Input: part model. Units: mm. Frame: model coordinates. A direction names the side the tool comes from. Give positions to 0.01 mm unless a question says otherwise; leave off trailing zeros. Loops run counter-clockwise (first coordinate to the right, second up) from the corner with the lowest first, then second, coordinate; pieces in that order, holes last.
Autodesk Inventor part; units mm, degrees
ref_plane "YZ Plane" through (0, 0, 0) normal (1, 0, 0) x (0, 1, 0)
ref_plane "XZ Plane" through (0, 0, 0) normal (0, 1, 0) x (-1, 0, 0)
ref_plane "XY Plane" through (0, 0, 0) normal (0, 0, 1) x (1, 0, 0)
sketch "Sketch1" plane through (0, 0, 0) normal (0, 0, 1) x (1, 0, 0)
  line L0 (177.8, -0.9299) -> (0, -0.9299)
  line L1 (175.895, 75.2701) -> (177.8, 75.2701)
  line L2 (172.72, 5.08) -> (172.72, 72.0951)
  arc A0 (175.895, 75.2701) -> (172.72, 72.0951) centre (175.895, 72.0951) ccw
  line L3 (177.8, -0.9299) -> (177.8, 75.2701)
  line L4 (172.72, 5.08) -> (0, 5.08)
  line L5 (0, 5.08) -> (0, -0.9299)
  point P0 (172.72, 75.2701)
  dimension "d0" = 177.8
  dimension "d4" = 3.175
  dimension "d6" = 1.905
  dimension "d87" = 76.2
extrude "Extrusion1" add sketch "Sketch1" along normal blind 127
sketch "Sketch5" plane through (0, 5.08, 0) normal (0, 1, 0) x (1, 0, 0)
  line L0 (172.72, -127) -> (71.12, -127) construction
  line L1 (0, 0) -> (0, -127)
  line L2 (5.08, 0) -> (0, 0)
  arc A0 (0, 0) -> (66.04, -127) centre (174.6906, 10.1687) ccw
  line L3 (71.12, -127) -> (66.04, -127)
  line L4 (172.72, -127) -> (71.12, -127)
  line L5 (0, -127) -> (177.8, -127)
  line L6 (172.72, -127) -> (0, -127)
  dimension "d99" = 5.08
  dimension "d100" = 5.08
  dimension "d134" = 101.6
split body "Split2" sketch "Sketch5" result one side removed curves L2 A0 L3 removed pieces at (22.8484, 4.58, 104.8944)
sketch "Sketch10" plane through (172.72, 5.08, 127) normal (0, 1, 0) x (1, 0, 0)
  point P0 (-172.72, 127)
sketch "Sketch6" plane through (172.72, 5.08, 127) normal (0, 1, 0) x (1, 0, 0)
  line L0 (-106.68, 0) -> (-101.6, 0)
  line L1 (-172.72, 127) -> (0, 127)
  line L2 (-172.72, 127) -> (-167.64, 127)
  arc A0 (-172.72, 127) -> (-106.68, 0) centre (6.2398, 139.3887) ccw
  arc A1 (-167.64, 127) -> (-101.6, 0) centre (11.3198, 139.3887) ccw
  dimension "d135" = 5.08
extrude "Extrusion3" add sketch "Sketch6" along normal blind 76.2
hole "Hole2" at (177.8, 12.5964, 5.838) direction (-1, 0, 0) diameter 4 end through all
fillet "Fillet2" radius 3.175 1 edges at (24.8837, 81.28, 70.3725)
properties part number "Intake Back Panel Middle" material "ABS Plastic"
(1) Cut plane A-A (y = 25.5). Return the cut outline in (x, z).
Values follow:
outline: (0, 0) - (5.08, 0) arc R179.39 cw to (71.12, 127) - (66.04, 127) arc R179.39 ccw to start; (172.72, 0) - (177.8, 0) - (177.8, 127) - (172.72, 127) - close
(2) Ray query, probe 1 along Y at (x, z) = (14.5, 10); probe 2 along X at (y, z) = (47, 42); probe 3 along X at (y, z) = (30, 116.5). Return the intervals inside material, ascending.
Values follow:
probe 1: y = -0.93 to 5.08
probe 2: x = 8.02 to 13.1, 172.72 to 177.8
probe 3: x = 54.19 to 59.27, 172.72 to 177.8
(3) Reachability of faces 1 (the flat face through (90, -0.93, 63)), 2 (the cylindrical face through (20.282, 42.647, 71.286)), 3 (the flat face through (172.72, 38, 63)), 4 (the cylindrical face through (25.362, 41.081, 71.286)), 5 (the cylindrical face through (19.92, 2.03, 71.48)) from +Z, -Z, +X, -X, +Y, -Y: full face, straight path, thin tool, end or side. Return the list, or none.
Values follow:
face 1: +Z, -Z, +X, -X, -Y
face 2: +Z, -X, +Y
face 3: +Z, -Z, +Y
face 4: -Z, +Y
face 5: +Z, -X, +Y, -Y
(4) Pin query (flat end, axial travel): pin 1 Ø5 at (x, y) = (29, 19.5) entering from +Z; pin 2 Ø1 at (x, z) = (176.5, 81.5) entering from +Y; pin 3 Ø1 at (x, z) = (48.5, 32) entering from +Y; pin 4 Ø2.5 at (y, z) = (12.6, 5.84) entering from +X. Return the tip coordinate at first contact, or that it passes through.
Values follow:
pin 1: stops at z = 89.77
pin 2: stops at y = 75.27
pin 3: stops at y = 5.08
pin 4: passes through
(5) Mould query, pull axis Y, two halves, no side actions, for faces 6 (the flat face through (88, 3, 0)), 7 (the flat face through (90, 5.08, 63)), 8 (the cylindrical face through (175.22, 13.81, 7.43)). Classes: +Y half, -Y half, draft (parallel to the pull), parting line (faces both ways), or undercut.
Values follow:
face 6: draft
face 7: +Y half
face 8: undercut
(6) Cut plane B-B (x = 93). Return the cut outline in (y, z), and give its area (3 significant figures).
Values follow:
outline: (-0.93, 0) - (5.08, 0) - (5.08, 127) - (-0.93, 127) - close
area: 763 mm2
